```python
from build123d import *

# Parameters (mm, degrees)
BOSS_EXTRUDE1_DEPTH = 26.9875
SKETCH2_W           = 41.275
SKETCH2_H           = 20.6375
CUT_EXTRUDE1_DEPTH  = 64.5
SKETCH3_R           = 3.49885
CUT_EXTRUDE2_DEPTH  = 27.9875
FILLET1_R           = 2.38
FILLET2_R           = 2.38
SKETCH5_R           = 3.96875
CUT_EXTRUDE3_DEPTH  = 43.979079107
CUT_EXTRUDE4_DEPTH  = 43.979079107
SKETCH7_W           = 279.4
SKETCH7_H           = 449.58
BOSS_EXTRUDE2_DEPTH = 6.35
SKETCH11_W          = 22.404322508
SKETCH11_H          = 449.427276574
BOSS_EXTRUDE3_DEPTH = 38.1
CUT_EXTRUDE6_DEPTH  = 152.6075


with BuildPart() as part:
    # Sketch1 → Boss-Extrude1 (new body)
    with BuildSketch(Plane.XY):
        Polygon((-3.175, 19.685), (-34.925, -43.815), (9.525, -43.815), (9.525, 19.685), align=None)
    extrude(amount=BOSS_EXTRUDE1_DEPTH)

    # Sketch2 → Cut-Extrude1 (cut, through all)
    with BuildSketch(Plane(origin=(0, 19.685, 0), x_dir=(1, 0, 0), z_dir=(0, 1, 0))):
        with Locations((-14.2875, -13.49375)):
            Rectangle(SKETCH2_W, SKETCH2_H)
    extrude(amount=-CUT_EXTRUDE1_DEPTH, mode=Mode.SUBTRACT)

    # Sketch3 → Cut-Extrude2 (cut, through all)
    with BuildSketch(Plane.XY.offset(26.9875)):
        with Locations((-26.965492708, -39.543722561)):
            Circle(SKETCH3_R)
    extrude(amount=-CUT_EXTRUDE2_DEPTH, mode=Mode.SUBTRACT)

    # Fillet1
    fillet1_edges = [part.edges().sort_by_distance(p)[0] for p in [
        (9.525, -12.065, 26.9875),
        (9.525, -12.065, 0),
    ]]
    fillet(fillet1_edges, radius=FILLET1_R)

    # Fillet2
    fillet2_edges = [part.edges().sort_by_distance(p)[0] for p in [
        (-34.925, -43.815, 1.5875),
        (-34.925, -43.815, 25.4),
    ]]
    fillet(fillet2_edges, radius=FILLET2_R)

    # Sketch5 → Cut-Extrude3 (cut, through all)
    with BuildSketch(Plane(origin=(9.525, 0, 0), x_dir=(0, 0, -1), z_dir=(1, 0, 0))):
        with Locations((-12.488615689, 8.5725)):
            Circle(SKETCH5_R)
    extrude(amount=-CUT_EXTRUDE3_DEPTH, mode=Mode.SUBTRACT)

    # Sketch6 → Cut-Extrude4 (cut, through all)
    with BuildSketch(Plane(origin=(9.525, 0, 0), x_dir=(0, 0, -1), z_dir=(1, 0, 0))):
        with BuildLine():
            Line((-8.73125, -43.815), (-18.25625, -43.815))
            Line((-18.25625, -43.815), (-18.25625, -32.7025))
            ThreePointArc((-18.25625, -32.7025), (-13.49375, -27.94), (-8.73125, -32.7025))
            Line((-8.73125, -32.7025), (-8.73125, -43.815))
        make_face()
    extrude(amount=-CUT_EXTRUDE4_DEPTH, mode=Mode.SUBTRACT)

    # Sketch7 → Boss-Extrude2 (add)
    with BuildSketch(Plane(origin=(-10.414, 5.207, 0), x_dir=(0, 0, 1), z_dir=(-0.894427191, 0.447213595, 0))):
        with Locations((12.7, 189.707658697)):
            Rectangle(SKETCH7_W, SKETCH7_H)
    extrude(amount=BOSS_EXTRUDE2_DEPTH)

    # Sketch11 → Boss-Extrude3 (add)
    with BuildSketch(Plane(origin=(-10.414, 5.207, 0), x_dir=(0, 0, -1), z_dir=(0.894427191, -0.447213595, 0))):
        with Locations((-13.405338746, 189.78402041)):
            Rectangle(SKETCH11_W, SKETCH11_H)
    extrude(amount=BOSS_EXTRUDE3_DEPTH)

    # Sketch13 → Cut-Extrude6 (cut, through all)
    with BuildSketch(Plane.XY.offset(24.6075)):
        Polygon((174.954988272, 375.944976544), (9.525, -40.109189943), (209.032664249, 358.906138556), align=None)
    extrude(amount=-CUT_EXTRUDE6_DEPTH, mode=Mode.SUBTRACT)


solid = part.part
```
Source: CAD feature listing. Evaluate the final solid. Frame: model axes, mm. A direction names the side the tool comes from. Give positions to 0.01 mm unless a question says otherwise; leave off trailing zeros. Loops run counter-clockwise (first coordinate to the right, second up) from the corner with the lowest first, then second, coordinate; pieces in that order, holes last. Notation, with made-up numbers: (55, -12.5) -> (111, -12.5) arc R27 ccw to (111, 14.5) -> close; hole circle Ø4 at (83, 68). An arc over 180 degrees is marked (long way). Use a Markdown table: item, result. Add a question column.
(1) Section query B-B (x = 109). Output: boundary loops of the cut face in (y, z) (1 decimal).
(2) Pull-direction query (Z, two-part tool) for faces 5 (the face through (-7, -43.815, 25)), 6 (the face through (65, 123, 2.203)), 7 (the face through (-18, -37, 3.175)); classes: +Z half, -Z half, draft (parallel to the pull), parting line (faces both ways), or undercut.
(3) Section query A-A (y = 37). Output: boundary loops of the cut face in (x, z), then the cut area to 3 significant figures.
(4) First-contact query: pin 1 Ø1.1 at (x, z) = (6, 0.5) entering from +Y; pin 2 Ø1.6 at (x, y) = (8.5, -42.5) entering from -Z; pin 3 Ø5.5 at (x, y) = (-5, -38) entering from -Z; pin 4 Ø6.5 at (x, y) = (-26.97, -39.54) entering from -Z. Flat tips, straight axial feed; report the tip coordinate or a pass-through.
(5) Section query C-C (z = -76). Output: boundary loops of the cut face in (x, y), then the cut area to 3 significant figures.
(6) Access query for faces 1 (the face through (-18, -37, 23.812)), 2 (the face through (-9, -19, 26.988)), 3 (the face through (-9, -19, 0)), 4 (the face through (70, 173, -127)). Directions: +Z, -Z, +X, -X, +Y, -Y. A direction counts if a zero-diameter tool reaches every point of the face in a straight line with its end or side. Return the directions, or none.
(7) Ray query, line 1 (Z direction, x = 122, y = 267); line 2 (Y direction, x = -15.5, z = 6); line 3 (X direction, y = 319.5, z = 83). Return the intervals inside material, ascending.
Checked values:
| question | item | result |
|---|---|---|
| 1 | outline | (210.1, 2.2) -> (244, 2.2) -> (244, -127) -> (258.2, -127) -> (258.2, 152.4) -> (244, 152.4) -> (244, 24.6) -> (210.1, 24.6) -> close |
| 2 | face 5 | draft |
| 2 | face 6 | -Z half |
| 2 | face 7 | undercut |
| 3 | outline | (-1.62, -127) -> (5.48, -127) -> (5.48, 2.2) -> (40.18, 2.2) -> (40.18, 24.61) -> (5.48, 24.61) -> (5.48, 152.4) -> (-1.62, 152.4) -> close |
| 3 | area | 2,760 mm^2 |
| 4 | pin 1 | y = 53.33 |
| 4 | pin 2 | z = 0.07 |
| 4 | pin 3 | z = 0 |
| 4 | pin 4 | through |
| 5 | outline | (-31.78, -23.33) -> (-26.1, -26.17) -> (174.95, 375.94) -> (169.28, 378.78) -> close |
| 5 | area | 2,850 mm^2 |
| 6 | face 1 | -X, -Y |
| 6 | face 2 | +Z, +X, -Y |
| 6 | face 3 | -Z, +X, -Y |
| 6 | face 4 | -Z, +X, -X, +Y, -Y |
| 7 | line 1 | 2.2 to 24.61 |
| 7 | line 2 | -31.3 to 9.23 |
| 7 | line 3 | 139.63 to 146.73 |
